from build123d import *

# Parameters (mm, degrees)
F0_W      = 38.1
F0_H      = 38.1
F1_DEPTH  = 38.1
F6_DEPTH  = 38.1
F8_DEPTH  = 38.1
F9_W      = 25.4
F9_H      = 7.62
F10_DEPTH = 38.1


with BuildPart() as f1:
    # F0 (on Front) → F1 (new body)
    with BuildSketch(Plane.XZ):
        with Locations((19.05, 19.05)):
            Rectangle(F0_W, F0_H)
    extrude(amount=F1_DEPTH)

    # F5 (on offset) → F6 (cut)
    with BuildSketch(Plane.YZ.offset(38.1)):
        Polygon((-31.75, 0), (-38.1, 38.1), (-38.1, 0), align=None)
        Polygon((-11.43, 11.71486), (-6.35, 38.1), (-31.75, 38.1), (-26.67, 11.752735), (-21.59, 28.575), (-16.51, 28.575), align=None)
        Polygon((-25.4, 0), (-12.7, 0), (-19.05, 15.875), align=None)
        Polygon((-6.35, 0), (0, 0), (0, 38.1), align=None)
    extrude(amount=-F6_DEPTH, mode=Mode.SUBTRACT)

    # F7 (on offset) → F8 (cut)
    with BuildSketch(Plane.XZ.offset(38.1)):
        Polygon((0, 38.1), (0, 0), (6.35, 38.1), align=None)
        Polygon((25.4, 38.1), (12.7, 38.1), (19.05, 22.225), align=None)
        Polygon((31.75, 38.1), (38.1, 0), (38.1, 38.1), align=None)
        Polygon((11.43, 20.18944), (6.35, 0), (31.75, 0), (26.67, 18.943178), (21.59, 9.525), (16.51, 9.525), align=None)
    extrude(amount=-F8_DEPTH, mode=Mode.SUBTRACT)

    # F9 (on offset) → F10 (cut)
    with BuildSketch(Plane.XY.offset(38.1)):
        with Locations((25.4, -11.43)):
            Rectangle(F9_W, F9_H)
        with Locations((12.7, -26.67)):
            Rectangle(F9_W, F9_H)
    extrude(amount=-F10_DEPTH, mode=Mode.SUBTRACT)


solid = f1.part
Build history of the part. All positions in model axes, mm. A direction names the side the tool comes from. Coordinates: 2 decimals unless noted, no trailing zeros. Write each loop counter-clockwise with the first axis right and the second up, starting at its lowest first coordinate (ties: lowest second). Pieces come first, ordered by that corner, then holes. Notation, with made-up numbers: (45, 15.25) -> (80, 15.25) arc R18 cw to (80, 31.25) -> close; hole circle Ø11 at (-2, 11). An arc over 180 degrees is marked (long way). Use CSV: the item, a comma, the result in double quotes. Start each with the question number.
Q1. Pull direction X, two halves, no side cores. Call faces 1 (the flat face through (6, -21, 11)), 2 (the flat face through (3.13, -9.05, 18.78)), 3 (the flat face through (13.44, -5.89, 15.97)): released by +X, released by -X, zero draft, split by the parting line, or undercut.
Q2. Cut at B-B, the plane z = 28. List the corners of the cut face in (x, y).
Q3. Cut at A-A, the plane x = 3.5. List the corners of the cut face in (y, z) (3 decimals).
Q4. 3-axis set-ups, long thin cutter, end or side, ignore diameter. For faces 4 (the flat face through (27.071, -15.884, 26.497)), 5 (the flat face through (19, -16, 9.525)), 6 (the flat face through (13, -30.48, 19)), 7 (the flat face through (15.83, -33.5, 30.27)): which of +Z, -Z, +X, -X, +Y, -Y reach the whole face in a straight line?
Q5. Flat gauge pins, fed straight in: pin 1 Ø6 at (y, z) = (-7.5, 34) entering from +X; pin 2 Ø1.4 at (y, z) = (-29, 22) entering from -X; pin 3 Ø14.5 at (x, z) = (21, 13.5) entering from +Y; pin 4 Ø12 at (x, y) = (6.5, -27.5) entering from +Z. Where does each tip first touch, or does it go through?
Q6. Cut at C-C, the plane x = 24. List the corners of the cut face in (y, z) (3 decimals), then the cut area to 3 significant figures.
Q7. Drill centre lines: probe 1 along Y at (x, z) = (22.5, 12); probe 2 along Y at (x, z) = (19, 10); probe 3 along Y at (x, z) = (26, 20.5). Where is each one in solid material? Low to high.
Checked values:
1,face 1,"zero draft"
1,face 2,"released by -X"
1,face 3,"undercut"
2,outline,"(4.67, -36.42) -> (16.74, -36.42) -> (16.74, -30.48) -> (4.67, -30.48) -> close; (4.67, -21.76) -> (16.74, -21.76) -> (16.74, -16.34) -> (4.67, -16.34) -> close; (4.67, -8.29) -> (12.7, -8.29) -> (12.7, -7.62) -> (16.74, -7.62) -> (16.74, -1.68) -> (4.67, -1.68) -> close; (21.36, -36.42) -> (33.43, -36.42) -> (33.43, -29.8) -> (25.4, -29.8) -> (25.4, -30.48) -> (21.36, -30.48) -> close; (21.36, -21.76) -> (33.43, -21.76) -> (33.43, -16.34) -> (21.36, -16.34) -> close; (21.36, -7.62) -> (33.43, -7.62) -> (33.43, -1.68) -> (21.36, -1.68) -> close"
3,outline,"(-35.25, 21) -> (-31.75, 0) -> (-30.48, 0) -> (-30.48, 21) -> close; (-22.86, 6.35) -> (-19.05, 15.875) -> (-12.7, 0) -> (-6.35, 0) -> (-2.85, 21) -> (-9.642, 21) -> (-11.43, 11.715) -> (-14.228, 21) -> (-22.86, 21) -> close"
4,face 4,"+Z, +X, -X"
4,face 5,"-Z, +Y, -Y"
4,face 6,"+Z, -Z, -X"
4,face 7,"+Z, +Y, -Y"
5,pin 1,"stops at x = 32.93"
5,pin 2,"stops at x = 25.4"
5,pin 3,"stops at y = -2.89"
5,pin 4,"stops at z = 38.1"
6,outline,"(-37.517, 34.6) -> (-34.082, 13.993) -> (-30.48, 13.993) -> (-30.48, 31.513) -> (-31.075, 34.6) -> close; (-22.86, 13.993) -> (-19.803, 13.993) -> (-19.05, 15.875) -> (-18.297, 13.993) -> (-15.24, 13.993) -> (-15.24, 24.36) -> (-16.51, 28.575) -> (-21.59, 28.575) -> (-22.86, 24.369) -> close; (-7.62, 13.993) -> (-4.018, 13.993) -> (-0.583, 34.6) -> (-7.024, 34.6) -> (-7.62, 31.504) -> close"
6,area,"322 mm²"
7,probe 1,"y = -33.75 to -30.48, -22.86 to -20.6, -17.5 to -15.24, -7.62 to -4.35"
7,probe 2,"y = -33.42 to -30.48, -22.86 to -21.4, -16.7 to -15.24, -7.62 to -4.68"
7,probe 3,"y = -35.17 to -28.36, -24.03 to -15.24, -7.62 to -2.93"
